Design review of the part built by this model. Coordinates are the model's own, in mm. A direction names the side the tool comes from. Round coordinates to 2 decimals unless told otherwise and drop trailing zeros. Write each loop counter-clockwise with the first axis right and the second up, starting at its lowest first coordinate (ties: lowest second). Pieces come first, ordered by that corner, then holes. Notation, with made-up numbers: (68.25, 17.5) -> (117.25, 17.5) arc R16 ccw to (117.25, 46.5) -> close; hole circle Ø6 at (39.5, 24.25). An arc over 180 degrees is marked (long way). Write item = value, one per line. Start each with the question number.
Item 1: Mouldability with a two-part tool opening along Y and no side actions: class faces 3 (the flat face through (30, 5, 20)), 4 (the flat face through (11.25, 0.35, 40)), 5 (the flat face through (-4.45, -10.06, 20.28)) as released by +Y, released by -Y, zero draft, split by the parting line, or undercut.
Item 2: Add section C-C, the plane x = 12. State the section outline as (y, z) points, then the cut area to 3 significant figures.
Item 3: For pin 1 Ø12 at (x, y) = (-11, 0) entering from +Z; pin 2 Ø8.5 at (x, z) = (29, 11) entering from -Y; pin 3 Ø5.5 at (x, z) = (28.5, 12) entering from +Y; pin 4 Ø5 at (y, z) = (-13, 28.5) entering from +X, all flat-tipped, find the tip position at first contact; note any pin that passes through.
Item 4: To check wall thickness, follow L1, parallel to Y at x = 9, z = 33; L2, parallel to Y at x = 1, z = 30; L3, parallel to Y at x = 25.5, z = 9.5. State the ranges of each line that lie inside material, in increasing order.
Item 5: Add section B-B, the plane y = 19. State the section outline as (x, z) points.
Item 6: Add section A-A, the plane z = 20. State the section outline as (x, y) points, then the cut area to 3 significant figures.
Item 7: Machinability: for faces 1 (the flat face through (5.522, -9.514, 20.28)), 2 (the flat face through (35, 0, 20)), which of the approach directions +Z, -Z, +X, -X, +Y, -Y give a long, thin tool a straight path to every point of the face, cutting with its end or side? Answer none if there is none.
from build123d import *

# Parameters (mm, degrees)
F1_DEPTH = 40
F3_DEPTH = 50


with BuildPart() as f1:
    # F0 (on Top) → F1 (new body)
    with BuildSketch(Plane.XY):
        with BuildLine():
            Line((35, 5), (24.494897, 5))
            ThreePointArc((24.494897, 5), (-25, 0), (24.494897, -5))
            Line((24.494897, -5), (35, -5))
            Line((35, -5), (35, 5))
        make_face()
    extrude(amount=F1_DEPTH)

    # F2 (on face) → F3 (cut)
    with BuildSketch(Plane.XY.offset(40)):
        Polygon((-10.379426, -4.037681), (-8.623709, -7.047482), (-6.023843, -9.367426), (-2.834321, -10.770422), (0.632644, -11.119133), (4.037681, -10.379426), (7.047482, -8.623709), (9.367426, -6.023843), (10.770422, -2.834321), (11.119133, 0.632644), (10.379426, 4.037681), (8.623709, 7.047482), (6.023843, 9.367426), (2.834321, 10.770422), (-0.632644, 11.119133), (-4.037681, 10.379426), (-7.047482, 8.623709), (-9.367426, 6.023843), (-10.770422, 2.834321), (-11.119133, -0.632644), align=None)
    extrude(amount=-F3_DEPTH, mode=Mode.SUBTRACT)


solid = f1.part
Result set:
q1.face_3 = released by +Y
q1.face_4 = zero draft
q1.face_5 = undercut
q2.outline = (-21.93, 0) -> (21.93, 0) -> (21.93, 40) -> (-21.93, 40) -> close
q2.area = 1,750 mm²
q3.pin_1 = 40
q3.pin_2 = -5
q3.pin_3 = 5
q3.pin_4 = 22.69
q4.L1 = -23.32 to -6.44, 6.4 to 23.32
q4.L2 = -24.98 to -11.04, 10.95 to 24.98
q4.L3 = -5 to 5
q5.outline = (-16.25, 0) -> (16.25, 0) -> (16.25, 40) -> (-16.25, 40) -> close
q6.outline = (24.49, -5) -> (35, -5) -> (35, 5) -> (24.49, 5) arc R25 ccw (long way) to start; hole (-11.12, -0.63) -> (-10.38, -4.04) -> (-8.62, -7.05) -> (-6.02, -9.37) -> (-2.83, -10.77) -> (0.63, -11.12) -> (4.04, -10.38) -> (7.05, -8.62) -> (9.37, -6.02) -> (10.77, -2.83) -> (11.12, 0.63) -> (10.38, 4.04) -> (8.62, 7.05) -> (6.02, 9.37) -> (2.83, 10.77) -> (-0.63, 11.12) -> (-4.04, 10.38) -> (-7.05, 8.62) -> (-9.37, 6.02) -> (-10.77, 2.83) -> close
q6.area = 1,680 mm²
q7.face_1 = +Z, -Z
q7.face_2 = +Z, -Z, +X, +Y, -Y
